Verification items for the finished model (mm, model axes). A direction names the side the tool comes from. Give positions to 0.01 mm unless a question says otherwise; leave off trailing zeros. Loops run counter-clockwise (first coordinate to the right, second up) from the corner with the lowest first, then second, coordinate; pieces in that order, holes last. Notation, with made-up numbers: (32, 18.25) - (60, 18.25) arc R35 ccw to (60, 54.25) - close; hole circle Ø1 at (-30, 5). An arc over 180 degrees is marked (long way). One line per item, written item: value. Start each with the question number.
1. Access from +Z, -Z, +X, -X, +Y, -Y to the whole of each face (thin tool, end or side, straight path). Record for faces 1 (the flat face through (-66.992, 15.26, 5.767)), 2 (the flat face through (-15, 5, 29)), 3 (the flat face through (-77.3, 9.5, 16.3)), 4 (the flat face through (-22.5, 9, 29)).
2. Sectioned sample at B-B (x = -35). Record the cut outline in (y, z).
3. Sectioned sample at D-D (z = 3.5). Record the cut outline in (x, y).
4. Scan lines: L1, parallel to X at y = 6.25, z = 1; L2, parallel to X at y = 2.5, z = 11; L3, parallel to Y at x = -44.25, z = 3.5. Record each from-to range of solid material in increasing order. Write a range as [from, to].
5. Sectioned sample at C-C (z = 9). Record the cut outline in (x, y).
6. Mould release check, pull along X, two halves, no side actions. Record for faces 5 (the flat face through (0, 10, 6)), 6 (the flat face through (-32.5, 6, 3)), 7 (the flat face through (-8, 3, 22)): pulls with the +X half, pulls with the -X half, needs draft (parallel to the pull), parting line crosses it, or undercut.
7. Sectioned sample at A-A (y = 3.25). Record the cut outline in (x, z).
8. Gauge pin test, flat ends, axial feed: pin 1 (5 mm diameter, centred on y = 2.5, z = 8.5, fed in from +X); pin 2 (2 mm diameter, centred on x = -75, y = 4, fed in from +Z); pin 3 (2 mm diameter, centred on y = 14.5, z = 21.5, fed in from -X). Record the tip position at first contact, or that the pin passes through.
from build123d import *

# Parameters (mm, degrees)
BOSS_EXTRUDE1_DEPTH = 16
SKETCH2_W           = 15
SKETCH2_H           = 7.75
SKETCH2_W_2         = 12.5
CUT_EXTRUDE1_DEPTH  = 5
CUT_EXTRUDE4_DEPTH  = 13
SKETCH6_W           = 55
SKETCH6_H           = 5.5
CUT_EXTRUDE5_DEPTH  = 3
SKETCH7_W           = 15
SKETCH7_H           = 7
SKETCH7_H_2         = 3
BOSS_EXTRUDE2_DEPTH = 13.25
SKETCH8_R           = 2.5
CUT_EXTRUDE6_DEPTH  = 15.5
SKETCH9_R           = 1.75
CUT_EXTRUDE7_DEPTH  = 15
SKETCH11_R          = 1.75
BOSS_EXTRUDE3_DEPTH = 3
SKETCH12_W          = 3
SKETCH12_H          = 19.5
BOSS_EXTRUDE4_DEPTH = 6.5
SKETCH13_W          = 1
SKETCH13_H          = 1.5
SKETCH13_W_2        = 18.5
CUT_EXTRUDE9_DEPTH  = 22
CUT_EXTRUDE10_DEPTH = 1.5


with BuildPart() as part:
    # Sketch1 → Boss-Extrude1 (new body)
    with BuildSketch(Plane(origin=(0, 0, 0), x_dir=(1, 0, 0), z_dir=(0, 1, 0))):
        Polygon((0, 0), (-80, 0), (-80, -7.75), (-80, -10.75), (-70.5, -10.75), (-70.5, -22), (-74.75, -22), (-72.5, -25), (-72.5, -32.75), (-7.5, -32.75), (-7.5, -22), (-9.5, -22), (-9.5, -10.75), (0, -10.75), (0, -7.75), align=None)
    extrude(amount=BOSS_EXTRUDE1_DEPTH)

    # Sketch2 → Cut-Extrude1 (cut)
    with BuildSketch(Plane.XZ):
        with Locations((-65, 28.875)):
            Rectangle(SKETCH2_W, SKETCH2_H)
        with Locations((-73.75, 3.875)):
            Rectangle(SKETCH2_W_2, SKETCH2_H)
        with Locations((-15, 28.875)):
            Rectangle(SKETCH2_W, SKETCH2_H)
        with Locations((-6.25, 3.875)):
            Rectangle(SKETCH2_W_2, SKETCH2_H)
    extrude(amount=-CUT_EXTRUDE1_DEPTH, mode=Mode.SUBTRACT)

    # Sketch5 → Cut-Extrude4 (cut)
    with BuildSketch(Plane.XZ):
        Polygon((-67.5, 25), (-67.5, 7.75), (-67.5, 0), (-12.5, 0), (-12.5, 7.75), (-12.5, 25), (-22.5, 25), (-22.5, 32.75), (-57.5, 32.75), (-57.5, 25), align=None)
    extrude(amount=-CUT_EXTRUDE4_DEPTH, mode=Mode.SUBTRACT)

    # Sketch6 → Cut-Extrude5 (cut)
    with BuildSketch(Plane.XZ.offset(-13)):
        with Locations((-40, 9.75)):
            Rectangle(SKETCH6_W, SKETCH6_H)
    extrude(amount=-CUT_EXTRUDE5_DEPTH, mode=Mode.SUBTRACT)

    # Sketch7 → Boss-Extrude2 (add)
    with BuildSketch(Plane.XZ.offset(-13)):
        with Locations((-40, 3.5)):
            Rectangle(SKETCH7_W, SKETCH7_H)
        with Locations((-40, 14)):
            Rectangle(SKETCH7_W, SKETCH7_H_2)
    extrude(amount=BOSS_EXTRUDE2_DEPTH)

    # Sketch8 → Cut-Extrude6 (cut)
    with BuildSketch(Plane(origin=(0, 0, 0), x_dir=(-1, 0, 0), z_dir=(0, 0, -1))):
        with Locations((40, -0.25)):
            Circle(SKETCH8_R)
    extrude(amount=-CUT_EXTRUDE6_DEPTH, mode=Mode.SUBTRACT)

    # Sketch9 → Cut-Extrude7 (cut)
    with BuildSketch(Plane(origin=(-32.5, 0, 0), x_dir=(0, 0, -1), z_dir=(1, 0, 0))):
        with Locations((-3.5, 3.25)):
            Circle(SKETCH9_R)
    extrude(amount=-CUT_EXTRUDE7_DEPTH, mode=Mode.SUBTRACT)

    # Sketch11 → Boss-Extrude3 (add)
    with BuildSketch(Plane(origin=(0, 6.5, 0), x_dir=(-1, 0, 0), z_dir=(0, -1, 0))):
        Polygon((70.5, -10.75), (70.5, -22), (74.75, -22), (80, -22), (80, -10.75), align=None)
        with Locations((75.25, -16.375)):
            Circle(SKETCH11_R, mode=Mode.SUBTRACT)
        Polygon((7.5, -32.75), (7.5, -22), (9.5, -22), (9.5, -10.75), (0, -10.75), (0, -11.25), (-14, -11.25), (-14, -30.75), (0, -30.75), align=None)
        with Locations((4.75, -16.375)):
            Circle(SKETCH11_R, mode=Mode.SUBTRACT)
    extrude(amount=-BOSS_EXTRUDE3_DEPTH)

    # Sketch12 → Boss-Extrude4 (add)
    with BuildSketch(Plane(origin=(0, 9.5, 0), x_dir=(1, 0, 0), z_dir=(0, 1, 0))):
        with BuildLine():
            ThreePointArc((-75.25, -10.75), (-71.891242789, -12.141242789), (-70.5, -15.5))
            Line((-70.5, -15.5), (-70.5, -10.75))
            Line((-70.5, -10.75), (-75.25, -10.75))
        make_face()
        with BuildLine():
            Line((-74.75, -21.973610907), (-74.75, -22))
            Line((-74.75, -22), (-70.5, -22))
            Line((-70.5, -22), (-70.5, -17.25))
            ThreePointArc((-70.5, -17.25), (-71.718888277, -20.427066257), (-74.75, -21.973610907))
        make_face()
        with Locations((12.5, -21)):
            Rectangle(SKETCH12_W, SKETCH12_H)
        with BuildLine():
            Line((-7.5, -32.75), (-6.5, -32.483333333))
            Line((-6.5, -32.483333333), (-6.5, -21.122983346))
            Line((-6.5, -21.122983346), (-7.5, -21.122983346))
            ThreePointArc((-7.5, -21.122983346), (-8.970485754, -19.429449472), (-9.5, -17.25))
            Line((-9.5, -17.25), (-9.5, -22))
            Line((-9.5, -22), (-7.5, -22))
            Line((-7.5, -22), (-7.5, -32.75))
        make_face()
        with BuildLine():
            ThreePointArc((-9.5, -15.5), (-8.108757211, -12.141242789), (-4.75, -10.75))
            Line((-4.75, -10.75), (-9.5, -10.75))
            Line((-9.5, -10.75), (-9.5, -15.5))
        make_face()
    extrude(amount=BOSS_EXTRUDE4_DEPTH)

    # Sketch13 → Cut-Extrude9 (cut)
    with BuildSketch(Plane.XY.offset(32.75)):
        with Locations((11.5, 13.25)):
            Rectangle(SKETCH13_W, SKETCH13_H)
        with Locations((1.75, 13.25)):
            Rectangle(SKETCH13_W_2, SKETCH13_H)
    extrude(amount=-CUT_EXTRUDE9_DEPTH, mode=Mode.SUBTRACT)

    # Sketch14 → Cut-Extrude10 (cut)
    with BuildSketch(Plane(origin=(0, 16, 0), x_dir=(1, 0, 0), z_dir=(0, 1, 0))):
        Polygon((-4.75, -10.75), (-1.921572875, -10.75), (-10.171572875, -2.5), (-38.36287075, -2.5), (-66.554168625, -2.5), (-70.224250191, -6.170081566), (-70.224250191, -13.329918434), (-66.554168625, -17), (-16.554168625, -17), (-14.939672781, -18.614495844), (-14.939672781, -20.897737763), (-16.554168625, -22.512233607), (-67.954977352, -22.512233607), (-70.224250191, -24.781506445), (-70.224250191, -28.721602613), (-67.954977352, -30.990875451), (-6.5, -30.990875451), (-6.5, -28.990875451), (-67.126550228, -28.990875451), (-68.224250191, -27.893175488), (-68.224250191, -25.60993357), (-67.126550228, -24.512233607), (-15.7257415, -24.512233607), (-12.939672781, -21.726164888), (-12.939672781, -17.786068719), (-15.7257415, -15), (-65.7257415, -15), (-68.224250191, -12.50149131), (-68.224250191, -9.75), (-68.224250191, -6.99850869), (-65.7257415, -4.5), (-38.36287075, -4.5), (-11, -4.5), align=None)
    extrude(amount=-CUT_EXTRUDE10_DEPTH, mode=Mode.SUBTRACT)


solid = part.part
Results are:
1. face 1: +Y
1. face 2: +Z, +X, -X, -Y
1. face 3: -X, +Y
1. face 4: +Z, -Z, -Y
2. outline: (-0.25, 0) - (16, 0) - (16, 2.5) - (14.5, 2.5) - (14.5, 4.5) - (16, 4.5) - (16, 7) - (-0.25, 7) - close; (-0.25, 12.5) - (16, 12.5) - (16, 15) - (14.5, 15) - (14.5, 17) - (16, 17) - (16, 22.51) - (14.5, 22.51) - (14.5, 24.51) - (16, 24.51) - (16, 28.99) - (14.5, 28.99) - (14.5, 30.99) - (16, 30.99) - (16, 32.75) - (13, 32.75) - (13, 15.5) - (-0.25, 15.5) - close; hole circle Ø3.5 at (3.25, 3.5)
3. outline: (-80, 5) - (-67.5, 5) - (-67.5, 13) - (-47.5, 13) - (-47.5, 5) - (-32.5, 5) - (-32.5, 13) - (-12.5, 13) - (-12.5, 5) - (0, 5) - (0, 16) - (-9.17, 16) - (-9.17, 14.5) - (-67.55, 14.5) - (-67.55, 16) - (-80, 16) - close; (-47.5, -0.25) - (-42.5, -0.25) arc R2.5 cw to (-41.79, 1.5) - (-47.5, 1.5) - close; (-38.21, 1.5) arc R2.5 cw to (-37.5, -0.25) - (-32.5, -0.25) - (-32.5, 1.5) - close
4. L1: x = [-80, -67.5], [-47.5, -32.5], [-12.5, 0]
4. L2: x = [-70.5, -67.5], [-12.5, -9.5]
4. L3: y = [-0.25, 1.5], [5, 14.5]
5. outline: (-80, 0) - (-67.5, 0) - (-67.5, 16) - (-68.22, 16) - (-68.22, 14.5) - (-70.22, 14.5) - (-70.22, 16) - (-80, 16) - close; (-12.5, 0) - (0, 0) - (0, 16) - (-3.67, 16) - (-3.67, 14.5) - (-6.5, 14.5) - (-6.5, 16) - (-12.5, 16) - close
6. face 5: pulls with the +X half
6. face 6: undercut
6. face 7: needs draft
7. outline: (-80, 7.75) - (-67.5, 7.75) - (-67.5, 25) - (-72.5, 25) - (-74.75, 22) - (-70.5, 22) - (-70.5, 10.75) - (-80, 10.75) - close; (-47.5, 0) - (-32.5, 0) - (-32.5, 1.75) - (-47.5, 1.75) - close; (-47.5, 5.25) - (-32.5, 5.25) - (-32.5, 7) - (-47.5, 7) - close; (-47.5, 12.5) - (-32.5, 12.5) - (-32.5, 15.5) - (-47.5, 15.5) - close; (-12.5, 7.75) - (0, 7.75) - (0, 10.75) - (-9.5, 10.75) - (-9.5, 22) - (-7.5, 22) - (-7.5, 25) - (-12.5, 25) - close
8. pin 1: stops at x = 0
8. pin 2: stops at z = 23
8. pin 3: stops at x = -74.75
